Can you work these out from the model? Positions are in its coordinate system, mm. A direction names the side the tool comes from. Give positions to 0.01 mm unless a question says otherwise; leave off trailing zeros. Loops run counter-clockwise (first coordinate to the right, second up) from the corner with the lowest first, then second, coordinate; pieces in that order, holes last. Notation, with made-up numbers: (-22, 89) -> (-15, 89) arc R28 ccw to (-15, 110) -> close; hole circle Ø5 at (35, 63). An arc over 180 degrees is marked (long way). Return JSON: item names as keys, results as strings. Group by question number.
Q1. Suppose I cut it at B-B, the plane y = 110. Please give me the cut outline in (x, z), and give its area (3 significant figures).
Q2. Will these pins go through, and if not, where does the flat tip stop? pin 1 (8 mm diameter, centred on y = 172, z = -14, fed in from -X); pin 2 (12 mm diameter, centred on x = 992.5, y = 119, fed in from +Z); pin 3 (2 mm diameter, centred on y = 296, z = 59.5, fed in from -X).
Q3. Thinking about a two-plate mould opening in X: for faces 1 (the flat face through (-179, 152, -23.5)), 2 (the flat face through (-18, 152, -7.5)), 3 (the flat face through (1237.955, 274.65, -3.698)), 4 (the flat face through (-1237.955, 25.35, -3.698)), which applies, pulls with the +X half, pulls with the -X half, needs draft (parallel to the pull), parting line crosses it, or undercut?
Q4. Suppose I cut it at C-C, the plane x = -7.5. Please give me the cut outline in (y, z).
Q5. I need wall thicknesses on line 1 along X through (y, z) = (168.5, -14); line 2 along Y through (x, z) = (-289.5, 45.5); line 3 along Z through (x, y) = (1119, 93.5). Which ranges of each line are inside material? Lowest first, please. Write a range as [from, to].
Q6. Suppose I cut it at A-A, the plane z = 21.5. Please give me the cut outline in (x, y), and give its area (3 significant figures).
Q7. Which directions (+Z, -Z, +X, -X, +Y, -Y) give clear straight access to the entire face, cutting with the end or side of a thin tool? Please do faces 5 (the flat face through (1237.045, 24.65, -3.698)), 6 (the flat face through (-18, 7.5, 44)).
```python
from build123d import *

# Parameters (mm, degrees)
EXTRUDE_589_DEPTH = 7.5
SKETCH_2_W        = 2408.049034164
SKETCH_2_H        = 7.5
EXTRUDE_1_DEPTH   = 89
SKETCH_3_W        = 80
SKETCH_3_H        = 240
EXTRUDE_2_DEPTH   = 16


with BuildPart() as part:
    # 草图1 → Extrude 589 (new body)
    with BuildSketch(Plane.XY):
        Polygon((-1205, 0), (1205, 0), (1270, 50), (1270, 250), (1205, 300), (-1205, 300), (-1270, 250), (-1270, 50), align=None)
    extrude(amount=-EXTRUDE_589_DEPTH)

    # 草图2 → 凸台-拉伸1 (add)
    with BuildSketch(Plane.XY):
        with Locations((-0.975482918, 296.25)):
            Rectangle(SKETCH_2_W, SKETCH_2_H)
        with Locations((-0.975482918, 3.75)):
            Rectangle(SKETCH_2_W, SKETCH_2_H)
    extrude(amount=EXTRUDE_1_DEPTH)

    # 草图3 → 凸台-拉伸2 (add)
    with BuildSketch(Plane(origin=(0, 0, -7.5), x_dir=(-1, 0, 0), z_dir=(0, 0, -1))):
        with Locations((-580, 150)):
            Rectangle(SKETCH_3_W, SKETCH_3_H)
        with Locations((-180, 150)):
            Rectangle(SKETCH_3_W, SKETCH_3_H)
        with Locations((180, 150)):
            Rectangle(SKETCH_3_W, SKETCH_3_H)
        with Locations((580, 150)):
            Rectangle(SKETCH_3_W, SKETCH_3_H)
    extrude(amount=EXTRUDE_2_DEPTH)


solid = part.part
```
Ans:
{
 "1": {"outline": "(-1270, -7.5) -> (-620, -7.5) -> (-620, -23.5) -> (-540, -23.5) -> (-540, -7.5) -> (-220, -7.5) -> (-220, -23.5) -> (-140, -23.5) -> (-140, -7.5) -> (140, -7.5) -> (140, -23.5) -> (220, -23.5) -> (220, -7.5) -> (540, -7.5) -> (540, -23.5) -> (620, -23.5) -> (620, -7.5) -> (1270, -7.5) -> (1270, 0) -> (-1270, 0) -> close", "area": "24,200 mm^2"},
 "2": {"pin 1": "stops at x = -620", "pin 2": "stops at z = 0", "pin 3": "stops at x = -1205"},
 "3": {"face 1": "needs draft", "face 2": "undercut", "face 3": "pulls with the +X half", "face 4": "pulls with the -X half"},
 "4": {"outline": "(0, -7.5) -> (300, -7.5) -> (300, 89) -> (292.5, 89) -> (292.5, 0) -> (7.5, 0) -> (7.5, 89) -> (0, 89) -> close"},
 "5": {"line 1": "x = [-620, -540], [-220, -140], [140, 220], [540, 620]", "line 2": "y = [0, 7.5], [292.5, 300]", "line 3": "z = [-7.5, 0]"},
 "6": {"outline": "(-1205, 0) -> (1203.05, 0) -> (1203.05, 7.5) -> (-1205, 7.5) -> close; (-1205, 292.5) -> (1203.05, 292.5) -> (1203.05, 300) -> (-1205, 300) -> close", "area": "36,100 mm^2"},
 "7": {"face 5": "+Z, -Z, +X, -Y", "face 6": "+Z, +X, -X"}
}
